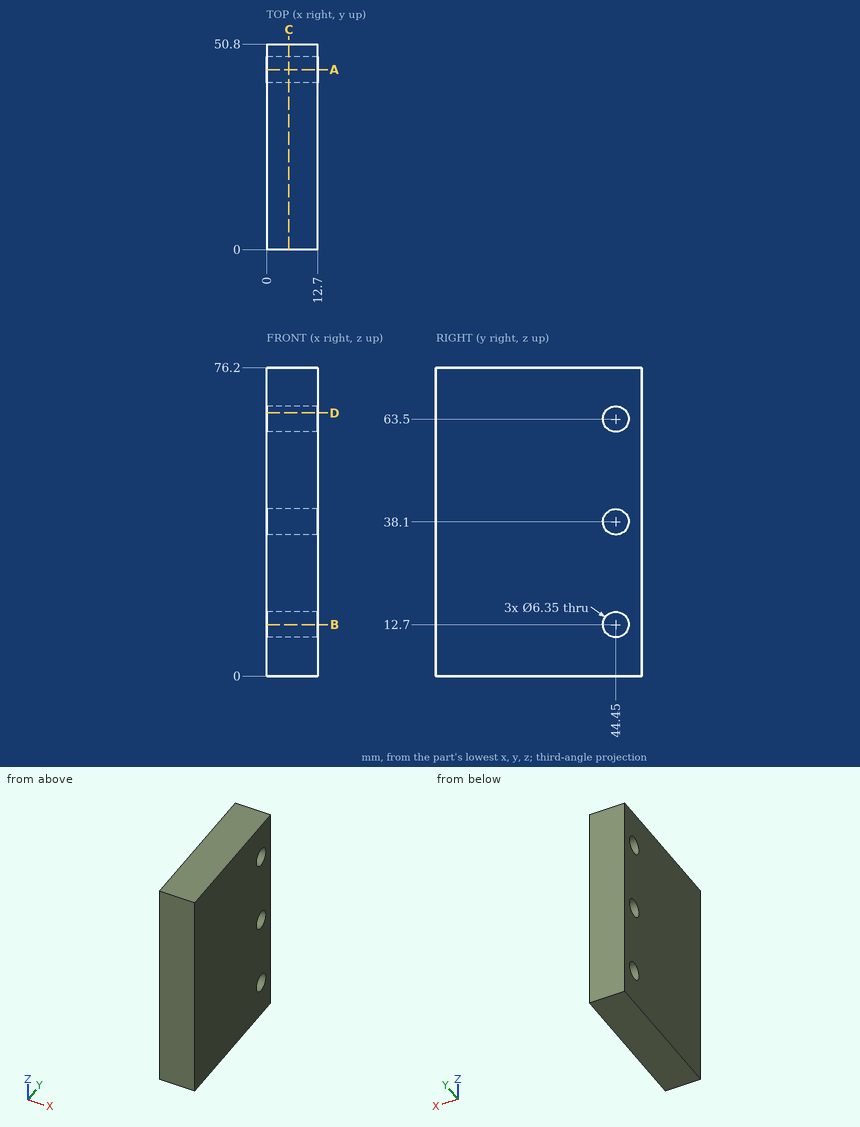
Input: dimensioned drawing with shaded views. Units: mm. Origin: part minimum x, y, z. Coordinates: 2 decimals unless noted, no trailing zeros. Order: outer loops, then holes, each group sorted by start corner. A loop starts at its lowest first (then second) coordinate and runs counter-clockwise, first axis right, second up. Notation, with made-up numbers: (52, 55.25) -> (109, 55.25) arc R22 cw to (109, 82.25) -> close; hole circle Ø4 at (-23, -25.75). An arc over 180 degrees is marked (long way). Answer in a Markdown table with one row per item.
Item 1: Section D-D on z = 65. Output: boundary loops of the cut face in (x, y), plus the area to 3 significant figures.
Return value:
| item | result |
|---|---|
| outline | (0, 0) -> (12.7, 0) -> (12.7, 41.65) -> (0, 41.65) -> close; (0, 47.25) -> (12.7, 47.25) -> (12.7, 50.8) -> (0, 50.8) -> close |
| area | 574 mm² |
Item 2: Section B-B on z = 12.7. Output: boundary loops of the cut face in (x, y) (3 decimals).
Return value:
| item | result |
|---|---|
| outline | (0, 0) -> (12.7, 0) -> (12.7, 41.275) -> (0, 41.275) -> close; (0, 47.625) -> (12.7, 47.625) -> (12.7, 50.8) -> (0, 50.8) -> close |
Item 3: Ray query, L1, parallel to Y at x = 8.25, z = 63.5 (3 decimals); L2, parallel to Z at x = 6, y = 46.5; L3, parallel to Z at x = 9.75, y = 44. Return the intervals inside material, ascending.
Return value:
| item | result |
|---|---|
| L1 | y = 0 to 41.275, 47.625 to 50.8 |
| L2 | z = 0 to 10.28, 15.12 to 35.68, 40.52 to 61.08, 65.92 to 76.2 |
| L3 | z = 0 to 9.56, 15.84 to 34.96, 41.24 to 60.36, 66.64 to 76.2 |
Item 4: Section A-A on y = 44.45. Output: boundary loops of the cut face in (x, z) (3 decimals).
Return value:
| item | result |
|---|---|
| outline | (0, 0) -> (12.7, 0) -> (12.7, 9.525) -> (0, 9.525) -> close; (0, 15.875) -> (12.7, 15.875) -> (12.7, 34.925) -> (0, 34.925) -> close; (0, 41.275) -> (12.7, 41.275) -> (12.7, 60.325) -> (0, 60.325) -> close; (0, 66.675) -> (12.7, 66.675) -> (12.7, 76.2) -> (0, 76.2) -> close |
Item 5: Section C-C on x = 5.5. Output: boundary loops of the cut face in (y, z) (3 decimals).
Return value:
| item | result |
|---|---|
| outline | (0, 0) -> (50.8, 0) -> (50.8, 76.2) -> (0, 76.2) -> close; hole circle Ø6.35 at (44.45, 12.7); hole circle Ø6.35 at (44.45, 38.1); hole circle Ø6.35 at (44.45, 63.5) |
